from build123d import *

# Parameters (mm, degrees)
F1_DEPTH  = 38.1
F2_W      = 6.35
F2_H      = 6.35
F3_DEPTH  = 57.15
F2_W_2    = 12.7
F4_DEPTH  = 19.05
F5_W      = 31.75
F5_H      = 6.35
F6_DEPTH  = 6.35
F7_W      = 31.75
F7_H      = 6.35
F8_DEPTH  = 6.35
F10_DEPTH = 25.4
F12_DEPTH = 25.4


with BuildPart() as f1:
    # F0 (on Right) → F1 (new body)
    with BuildSketch(Plane.YZ):
        with BuildLine():
            Line((-12.7, 0), (0, 0))
            Line((0, 0), (0, 12.7))
            Line((0, 12.7), (-3.175, 12.7))
            ThreePointArc((-3.175, 12.7), (-6.35, 9.525), (-9.525, 12.7))
            Line((-9.525, 12.7), (-12.7, 12.7))
            Line((-12.7, 12.7), (-12.7, 0))
        make_face()
        with BuildLine():
            Line((-3.175, 12.7), (0, 12.7))
            Line((0, 12.7), (0, 19.05))
            Line((0, 19.05), (-12.7, 19.05))
            Line((-12.7, 19.05), (-12.7, 12.7))
            Line((-12.7, 12.7), (-9.525, 12.7))
            ThreePointArc((-9.525, 12.7), (-6.35, 15.875), (-3.175, 12.7))
        make_face()
    extrude(amount=F1_DEPTH)

    # F2 (on face) → F3 (join)
    with BuildSketch(Plane(origin=(0, 0, 0), x_dir=(0, -1, 0), z_dir=(-1, 0, 0))):
        with Locations((9.525, 3.175)):
            Rectangle(F2_W, F2_H)
        with Locations((15.875, 3.175)):
            Rectangle(F2_W, F2_H)
    extrude(amount=-F3_DEPTH)

    # F2 (on face) → F4 (join)
    with BuildSketch(Plane(origin=(0, 0, 0), x_dir=(0, -1, 0), z_dir=(-1, 0, 0))):
        with Locations((12.7, 3.175)):
            Rectangle(F2_W_2, F2_H)
    extrude(amount=F4_DEPTH)

    # F5 (on face) → F6 (join)
    with BuildSketch(Plane(origin=(-19.05, 0, 0), x_dir=(0, -1, 0), z_dir=(-1, 0, 0))):
        with Locations((34.925, 3.175)):
            Rectangle(F5_W, F5_H)
        Polygon((60.985425, 14.896587), (50.8, 6.35), (50.8, 0), align=None)
    extrude(amount=-F6_DEPTH)

    # F7 (on face) → F8 (join)
    with BuildSketch(Plane.YZ.offset(57.15)):
        Polygon((-50.8, 0), (-50.8, 6.35), (-60.910088, 14.833371), align=None)
        with Locations((-34.925, 3.175)):
            Rectangle(F7_W, F7_H)
    extrude(amount=-F8_DEPTH)

    # F9 (on face) → F10 (cut)
    with BuildSketch(Plane(origin=(0, -17.862572, -21.287784), x_dir=(1, 0, 0), z_dir=(0, 0.642788, 0.766044))):
        Polygon((-15.875, -56.292887), (-19.05, -42.996759), (-19.05, -56.292887), align=None)
        Polygon((-12.7, -42.996759), (-15.875, -56.292887), (-12.7, -56.292887), align=None)
    extrude(amount=-F10_DEPTH, mode=Mode.SUBTRACT)

    # F11 (on face) → F12 (cut)
    with BuildSketch(Plane(origin=(0, -17.862572, -21.287784), x_dir=(1, 0, 0), z_dir=(0, 0.642788, 0.766044))):
        Polygon((57.15, -42.996759), (53.975, -56.194541), (57.15, -56.194541), align=None)
        Polygon((50.8, -56.194541), (53.975, -56.194541), (50.8, -42.996759), align=None)
    extrude(amount=-F12_DEPTH, mode=Mode.SUBTRACT)


solid = f1.part
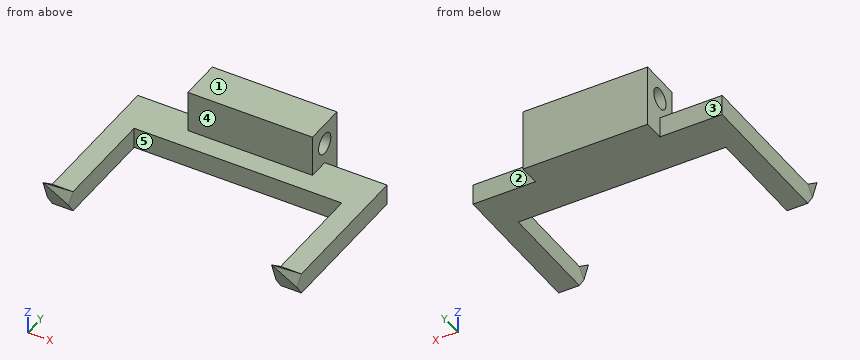
CAD build for the part. Positions are in the model's coordinates, mm. Face numbers are marked on the shaded views. A direction names the side the tool comes from. Round coordinates to 2 decimals unless told otherwise and drop trailing zeros. Order: outer loops, then holes, each group sorted by start corner. A loop starts at its lowest first (then second) coordinate and runs counter-clockwise, first axis right, second up. Notation, with made-up numbers: M 18.5,43 L 77.5,43 A24 ccw 77.5,70 Z; hole C 57,30.5 d8. An arc over 180 degrees is marked long. Use one line per item in the form item = value.
Q1. Saw through at C-C on z = 12.7. Give the cut face in (x, y) (3 decimals), then the cut area to 3 significant figures.
Recorded:
outline = M -16.691,-58.368 L -16.487,-59.484 L -15.263,-59.484 L -15.059,-58.368 Z; M 0,-12.7 L 38.1,-12.7 L 38.1,-9.525 L 0,-9.525 Z; M 0,-3.175 L 38.1,-3.175 L 38.1,0 L 0,0 Z; M 53.177,-58.368 L 53.377,-59.456 L 54.573,-59.456 L 54.773,-58.368 Z
area = 245 mm^2
Q2. Saw through at A-A on y = -36. Give the cut face in (x, z).
Recorded:
outline = M -19.05,0 L -12.7,0 L -12.7,6.35 L -19.05,6.35 Z; M 50.8,0 L 57.15,0 L 57.15,6.35 L 50.8,6.35 Z
Q3. Saw through at D-D on z = 5. Give the cut face in (x, y), then the cut area to 3 significant figures.
Recorded:
outline = M -19.05,-51.93 L -18.63,-54.22 L -13.12,-54.22 L -12.7,-51.93 L -12.7,-19.05 L 50.8,-19.05 L 50.8,-51.93 L 51.22,-54.21 L 56.73,-54.21 L 57.15,-51.93 L 57.15,-6.35 L 38.1,-6.35 L 38.1,0 L 0,0 L 0,-6.35 L -19.05,-6.35 Z
area = 1,650 mm^2
Q4. Flat gauge pins, fed straight in: P1, Ø4, axis at x = 8, z = 15, coming from the -Y side; P2, Ø5, axis at x = 49.5, z = 3.5, coming from the +Y side; P3, Ø8, axis at x = -4.5, z = 8.5, coming from the +Y side. Where does each tip first touch, or does it go through?
Recorded:
P1 = -12.7
P2 = -6.35
P3 = -6.35
Q5. Probe L1, parallel to X at y = -42.5, z = 3; L2, parallel to Z at x = 15, y = -6; L3, parallel to Z at x = 21, y = -15. List the from-to ranges inside material, lowest first.
Recorded:
L1 = -19.05 to -12.7, 50.8 to 57.15
L2 = 0 to 9.54, 15.86 to 19.05
L3 = 0 to 6.35
Q6. Which spindle directions (+Z, -Z, +X, -X, +Y, -Y) get a long thin tool onto all of the face, cutting with end or side? Do the marked faces 1, 2 and 3. Say none if no direction does.
Recorded:
face_1 = +Z, +X, -X, +Y, -Y
face_2 = +Z, -Z, +X, +Y
face_3 = +Z, -Z, -X, +Y
Q7. Two-plate mould, pull along X, no slides. Class the marked faces 4 and 5: +X half, -X half, draft (parallel to the pull), parting line (faces both ways), or undercut.
Recorded:
face_4 = draft
face_5 = undercut
Q8. Saw through at B-B on x = 28.5. Give the cut face in (y, z) (3 decimals).
Recorded:
outline = M -19.05,0 L 0,0 L 0,19.05 L -12.7,19.05 L -12.7,6.35 L -19.05,6.35 Z; hole C -6.35,12.7 d6.35
